Job drawing, mm, ordinate dimensions from the low corner. One solid piece. A direction names the side the tool comes from. Coordinates: 2 decimals unless noted, no trailing zeros. Order: outer loops, then holes, each group sorted by start corner. A loop starts at its lowest first (then second) coordinate and runs counter-clockwise, first axis right, second up. Notation, with made-up numbers: (3, -18.75) - (18, -18.75) arc R25 cw to (18, 12.25) - close; hole circle Ø5 at (-23.75, 43.25). An arc over 180 degrees is marked (long way). Use a Markdown table: item, result. Add a question column.
1) Saw through at D-D on y = 25. List the corners of the cut face in (x, z).
2) Wall check: L1, parallel to X at y = 29.5, z = 2.5; L2, parallel to Y at x = 10.25, z = 11; L3, parallel to Y at x = 1.6, z = 11.25. Give the ranges that are in metal, low to high. Write a range as [from, to].
3) Two-plate mould, pull along Y, no slides. Class the marked faces 1, 2 and 3: +Y half, -Y half, draft (parallel to the pull), parting line (faces both ways), or undercut.
4) Saw through at B-B on z = 20.5. List the corners of the cut face in (x, y).
5) Tool access for the marked faces 4 and 5: list every direction of +Z, -Z, +X, -X, +Y, -Y with a clear straight run to the whole face (end or side of a thin tool).
6) Saw through at C-C on y = 20. List the corners of the cut face in (x, z).
7) Saw through at A-A on x = 7. List the corners of the cut face in (y, z), then the cut area to 4 significant figures.
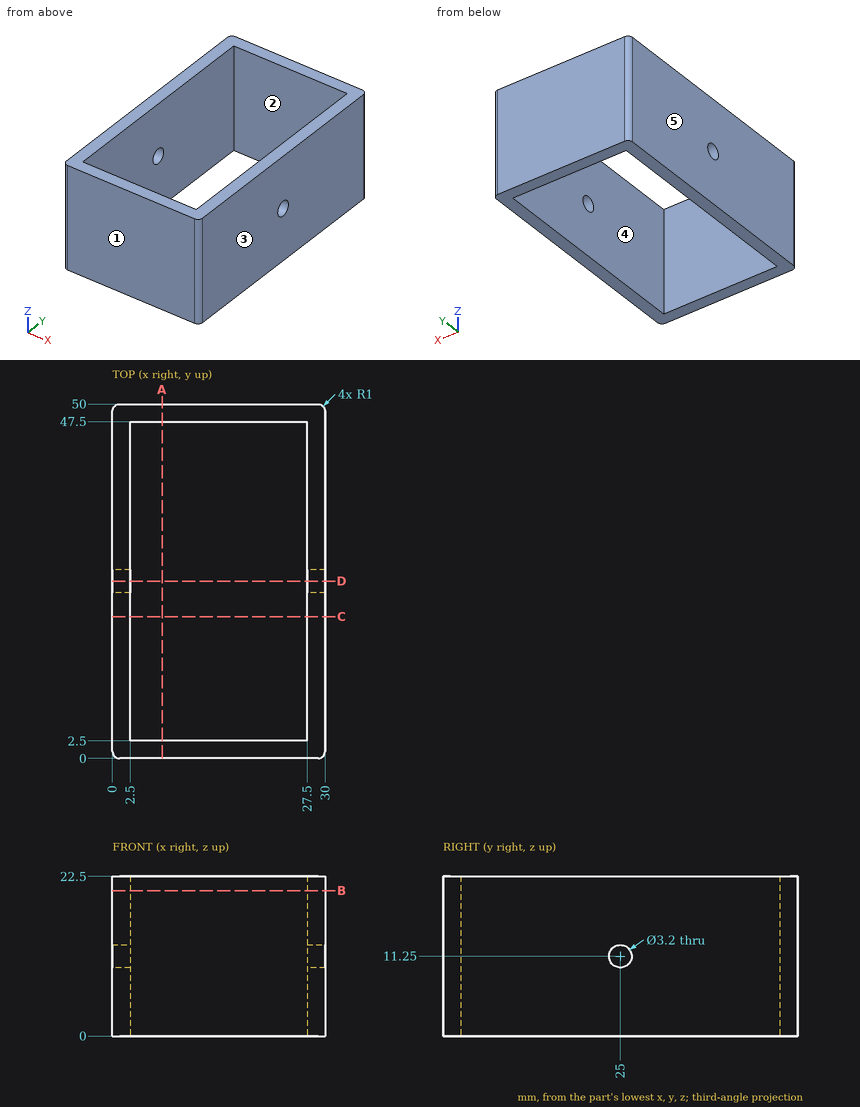
Results are:
| question | item | result |
|---|---|---|
| 1 | outline | (0, 0) - (2.5, 0) - (2.5, 9.65) - (0, 9.65) - close; (0, 12.85) - (2.5, 12.85) - (2.5, 22.5) - (0, 22.5) - close; (27.5, 0) - (30, 0) - (30, 9.65) - (27.5, 9.65) - close; (27.5, 12.85) - (30, 12.85) - (30, 22.5) - (27.5, 22.5) - close |
| 2 | L1 | [0, 2.5], [27.5, 30] |
| 2 | L2 | [0, 2.5], [47.5, 50] |
| 2 | L3 | [0, 23.4], [26.6, 50] |
| 3 | face 1 | -Y half |
| 3 | face 2 | undercut |
| 3 | face 3 | draft |
| 4 | outline | (0, 1) arc R1 ccw to (1, 0) - (29, 0) arc R1 ccw to (30, 1) - (30, 49) arc R1 ccw to (29, 50) - (1, 50) arc R1 ccw to (0, 49) - close; hole (2.5, 2.5) - (27.5, 2.5) - (27.5, 47.5) - (2.5, 47.5) - close |
| 5 | face 4 | +Z, -Z |
| 5 | face 5 | +Z, -Z, -X, +Y, -Y |
| 6 | outline | (0, 0) - (2.5, 0) - (2.5, 22.5) - (0, 22.5) - close; (27.5, 0) - (30, 0) - (30, 22.5) - (27.5, 22.5) - close |
| 7 | outline | (0, 0) - (2.5, 0) - (2.5, 22.5) - (0, 22.5) - close; (47.5, 0) - (50, 0) - (50, 22.5) - (47.5, 22.5) - close |
| 7 | area | 112.5 mm2 |
